Work out the finished part from the listing and answer in its coordinate system (mm). Face numbers are marked on the shaded views. A direction names the side the tool comes from. Coordinates: 2 decimals unless noted, no trailing zeros. Order: outer loops, then holes, each group sorted by start corner. A loop starts at its lowest first (then second) coordinate and runs counter-clockwise, first axis right, second up. Notation, with made-up numbers: (87.25, 28) -> (95.25, 28) arc R22 cw to (95.25, 45) -> close; hole circle Ø3 at (15.25, 84). An arc over 180 degrees is marked (long way). Write item = value, one per line. Start each with the question number.
Q1. Which of the six approach directions +Z, -Z, +X, -X, +Y, -Y give full straight-line access (tool end or side, diameter ignored) to the marked faces 4 and 5?
Q2. The part is cut by section A-A, the plane x = -28. Determine the outline of the cut face in (y, z), plus the area to 3 significant figures.
Q3. For a pull along Z with two mould halves and no side action, classify the marked faces 1, 2 and 3 as +Z half, -Z half, draft (parallel to the pull), parting line (faces both ways), or undercut.
Q4. The part is cut by section B-B, the plane z = 211.5. Determine the outline of the cut face in (x, y), plus the area to 3 significant figures.
Q5. Straight lines are drawn through the part: L1, parallel to Z at x = 36.5, y = -397; L2, parallel to Y at x = -6.5, z = 251; L3, parallel to Z at x = 14.5, y = -941. For each, find the intervals that lie inside material, in ascending order. Write a range as from..to.
Q6. The part is cut by section C-C, the plane y = -259. Determine the outline of the cut face in (x, z).
Q7. Flat-ended cylindrical pins translate along their axes: pin 1 (0.9 mm diameter, centred on x = -50.5, y = 53.5, fed in from +Z); pin 2 (7 mm diameter, centred on x = -12, y = 52.5, fed in from +Z); pin 3 (24 mm diameter, centred on y = 58, z = 475, fed in from +X). Find the tip coordinate at first contact, or state that the pin passes through.
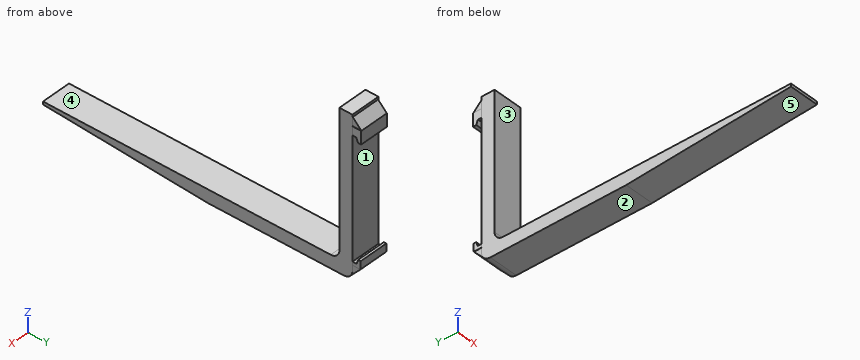
```python
from build123d import *

# Parameters (mm, degrees)
F1_DEPTH = 51.25
F2_R     = 30
F9_DEPTH = 50.8
F5_DEPTH = 50.8
F7_DEPTH = 50


with BuildPart() as f1:
    # F0 (on Right) → F1 (new body, symmetric)
    with BuildSketch(Plane.YZ):
        Polygon((-1025, -10), (-455, -45), (45, -45), (45, 496), (0, 496), (0, 0), (-1025, 0), align=None)
    extrude(amount=F1_DEPTH, both=True)

    # F2
    f2_edges = [f1.edges().sort_by_distance(p)[0] for p in [
        (0, 0, 0),
        (0, 45, -45),
    ]]
    fillet(f2_edges, radius=F2_R)

    # F3 (on Right) → F9 (join, symmetric)
    with BuildSketch(Plane.YZ):
        Polygon((45, 15), (45, 3), (72.5, 3), (72.5, 30), (64, 30), (59, 15), align=None)
    extrude(amount=F9_DEPTH, both=True)

    # F4 (on Right) → F5 (join, symmetric)
    with BuildSketch(Plane.YZ):
        Polygon((75, 457.5), (45, 457.5), (45, 428), (58, 428), (63.7, 413), (75, 413), align=None)
    extrude(amount=F5_DEPTH, both=True)

    # F6 (on Right) → F7 (join, symmetric)
    with BuildSketch(Plane.YZ):
        with BuildLine():
            Line((72.5, 3), (45, 3))
            Line((45, 3), (45, -15))
            ThreePointArc((45, -15), (42.9359111554, -25.9354866338), (37.0276754722, -35.3661855361))
            Line((37.0276754722, -35.3661855361), (72.5, 3))
        make_face()
        Polygon((75, 457.5), (45, 487.5), (45, 457.5), align=None)
    extrude(amount=F7_DEPTH, both=True)


solid = f1.part
```
Model answer:
q1.face_4 = +Z, +X, -X, -Y
q1.face_5 = -Z, +X, -X, -Y
q2.outline = (-1025, -10) -> (-455, -45) -> (15, -45) arc R30 ccw to (37.03, -35.37) -> (72.5, 3) -> (72.5, 30) -> (64, 30) -> (59, 15) -> (45, 15) -> (45, 428) -> (58, 428) -> (63.7, 413) -> (75, 413) -> (75, 457.5) -> (45, 487.5) -> (45, 496) -> (0, 496) -> (0, 30) arc R30 cw to (-30, 0) -> (-1025, 0) -> close
q2.area = 63,000 mm2
q3.face_1 = undercut
q3.face_2 = -Z half
q3.face_3 = draft
q4.outline = (-51.25, 0) -> (51.25, 0) -> (51.25, 45) -> (-51.25, 45) -> close
q4.area = 4,610 mm2
q5.L1 = -45..0
q5.L2 = 0..45
q5.L3 = -15.16..0
q6.outline = (-51.25, -45) -> (51.25, -45) -> (51.25, 0) -> (-51.25, 0) -> close
q7.pin_1 = 457.5
q7.pin_2 = 483.5
q7.pin_3 = 50
